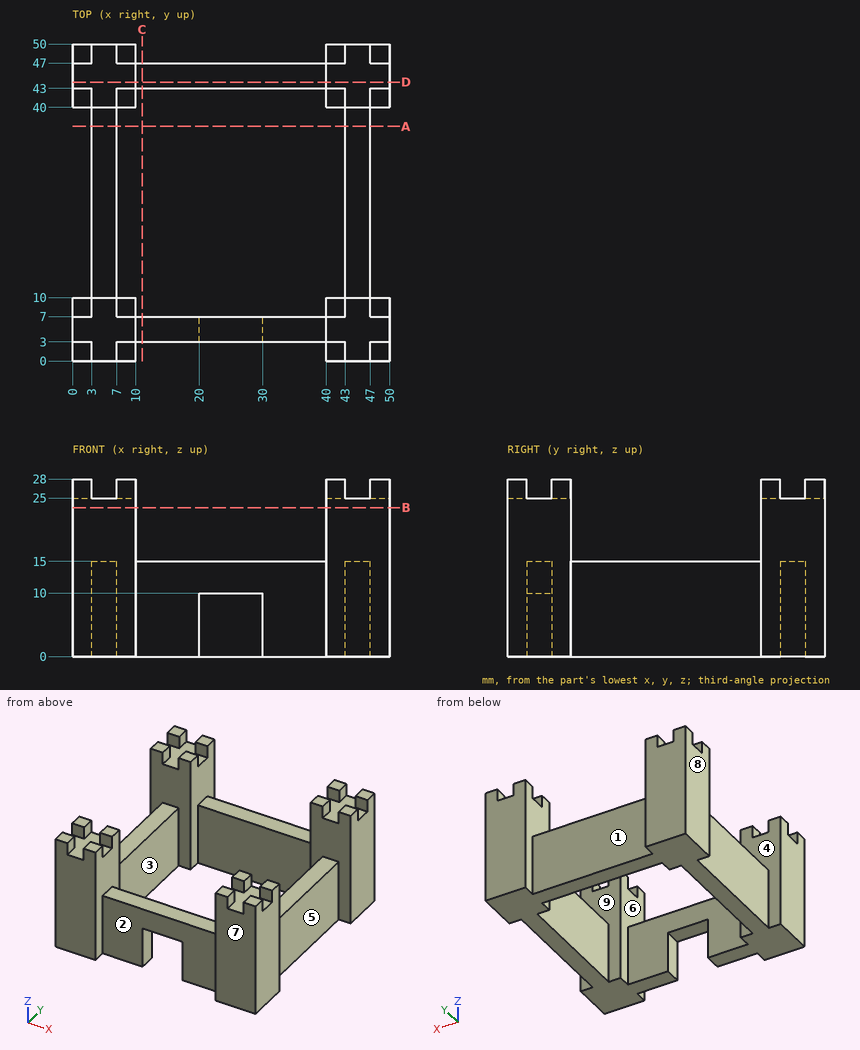
Check sheet for the drawn part. Datum: minimum x, y, z corner. Units: mm. A direction names the side the tool comes from. Coordinates: 2 decimals unless noted, no trailing zeros. Order: outer loops, then holes, each group sorted by start corner. A loop starts at its lowest first (then second) coordinate and runs counter-clockwise, first axis right, second up. Notation, with made-up numbers: M -31,1 L 17,1 A25 ccw 17,37 Z; hole C 84,88.5 d2. An arc over 180 degrees is marked long. One line per question, with ' | ' between items. Start each with the question number.
Item 1: Access from +Z, -Z, +X, -X, +Y, -Y to the whole of each face (thin tool, end or side, straight path). Record for the marked faces 1, 2, 3, 4 and 5.
Item 2: Material ranges on line 1 (X direction, y = 8, z = 26.25); line 2 (Y direction, x = 48, z = 2); line 3 (Y direction, x = 27, z = 13.5), recorded low to high.
Item 3: Gauge pin test, flat ends, axial feed: P1, Ø5, axis at x = 23.5, z = 13.5, coming from the -Y side; P2, Ø1.2, axis at x = 45.5, y = 30.5, coming from the +Z side; P3, Ø1, axis at x = 9, y = 11, coming from the +Z side; P4, Ø1.2, axis at x = 22.5, y = 4, coming from the -Z side. Record the tip position at first contact, or that the pin passes through.
Item 4: Sectioned sample at D-D on y = 44. Record the cut outline in (x, z).
Item 5: Mould release check, pull along Y, two halves, no side actions. Record for the marked faces 6, 7, 8 and 9: pulls with the +Y half, pulls with the -Y half, needs draft (parallel to the pull), parting line crosses it, or undercut.
Item 6: Sectioned sample at A-A on y = 37. Record the cut outline in (x, z).
Item 7: Sectioned sample at B-B on z = 23.5. Record the cut outline in (x, y).
Answer below:
1) face 1: +Z, -Z, +Y | face 2: +Z, -Z, -Y | face 3: +Z, -Z | face 4: +Z | face 5: +Z, -Z, +X
2) line 1: x = 0 to 3, 7 to 10, 40 to 43, 47 to 50 | line 2: y = 0 to 10, 40 to 50 | line 3: y = 3 to 7, 43 to 47
3) P1: stops at y = 3 | P2: stops at z = 15 | P3: passes through | P4: stops at z = 10
4) outline: M 0,0 L 50,0 L 50,25 L 40,25 L 40,15 L 10,15 L 10,25 L 0,25 Z
5) face 6: undercut | face 7: pulls with the -Y half | face 8: needs draft | face 9: undercut
6) outline: M 3,0 L 7,0 L 7,15 L 3,15 Z; M 43,0 L 47,0 L 47,15 L 43,15 Z
7) outline: M 0,0 L 10,0 L 10,10 L 0,10 Z; M 0,40 L 10,40 L 10,50 L 0,50 Z; M 40,0 L 50,0 L 50,10 L 40,10 Z; M 40,40 L 50,40 L 50,50 L 40,50 Z
